Geometry: see drawing. Coordinates: mm, zero at the bounding-box minimum. A direction names the side the tool comes from. Round coordinates to 2 decimals unless told otherwise and drop trailing zeros. Loops run counter-clockwise (first coordinate to the right, second up) from the corner with the lowest first, then second, coordinate; pieces in that order, holes last. Notation, with made-up numbers: (-24.75, 9) - (13.25, 9) arc R14 ccw to (13.25, 27) - close; hole circle Ø8 at (-20, 14). An arc over 180 degrees is marked (long way). One line per question, with ' | ' between items. Start each with the question number.
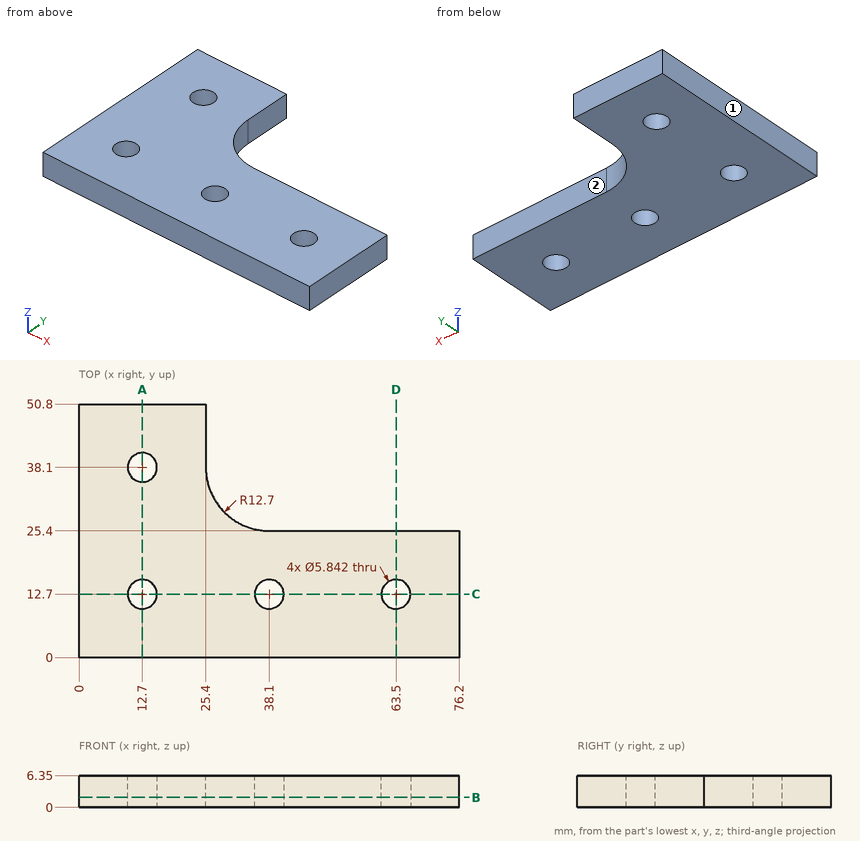
(1) Reachability of the marked faces 1 and 2 from +Z, -Z, +X, -X, +Y, -Y: full face, straight path, thin tool, end or side. Return the list, or none.
(2) Section D-D, the plane x = 63.5. Output: boundary loops of the cut face in (y, z).
(3) Line query: line 1 along Y through (x, z) = (12.7, 2.25); line 2 along Y through (x, z) = (38.1, 1.5); line 3 along X through (y, z) = (15, 2.5). Output: solid intervals per line, ascending. Write a range as from..to.
(4) Pin query (flat end, axial travel): P1, Ø3.5, axis at x = 63.5, y = 12.7, coming from the +Z side; P2, Ø10, axis at x = 60.5, y = 30, coming from the -Z side; P3, Ø1.5, axis at y = 28.5, z = 2, coming from the +X side. Return the tip coordinate at first contact, or that it passes through.
(5) Section C-C, the plane y = 12.7. Output: boundary loops of the cut face in (x, z).
(6) Section B-B, the plane z = 2. Output: boundary loops of the cut face in (x, y).
(7) Section A-A, the plane x = 12.7. Output: boundary loops of the cut face in (y, z), plus the area to 3 significant figures.
Derived:
1) face 1: +Z, -Z, -X, +Y, -Y | face 2: +Z, -Z, +X, +Y
2) outline: (0, 0) - (9.78, 0) - (9.78, 6.35) - (0, 6.35) - close; (15.62, 0) - (25.4, 0) - (25.4, 6.35) - (15.62, 6.35) - close
3) line 1: y = 0..9.78, 15.62..35.18, 41.02..50.8 | line 2: y = 0..9.78, 15.62..25.4 | line 3: x = 0..10.9, 14.5..36.3, 39.9..61.7, 65.3..76.2
4) P1: passes through | P2: stops at z = 0 | P3: stops at x = 30.74
5) outline: (0, 0) - (9.78, 0) - (9.78, 6.35) - (0, 6.35) - close; (15.62, 0) - (35.18, 0) - (35.18, 6.35) - (15.62, 6.35) - close; (41.02, 0) - (60.58, 0) - (60.58, 6.35) - (41.02, 6.35) - close; (66.42, 0) - (76.2, 0) - (76.2, 6.35) - (66.42, 6.35) - close
6) outline: (0, 0) - (76.2, 0) - (76.2, 25.4) - (38.1, 25.4) arc R12.7 cw to (25.4, 38.1) - (25.4, 50.8) - (0, 50.8) - close; hole circle Ø5.84 at (12.7, 12.7); hole circle Ø5.84 at (12.7, 38.1); hole circle Ø5.84 at (38.1, 12.7); hole circle Ø5.84 at (63.5, 12.7)
7) outline: (0, 0) - (9.78, 0) - (9.78, 6.35) - (0, 6.35) - close; (15.62, 0) - (35.18, 0) - (35.18, 6.35) - (15.62, 6.35) - close; (41.02, 0) - (50.8, 0) - (50.8, 6.35) - (41.02, 6.35) - close | area: 248 mm²
